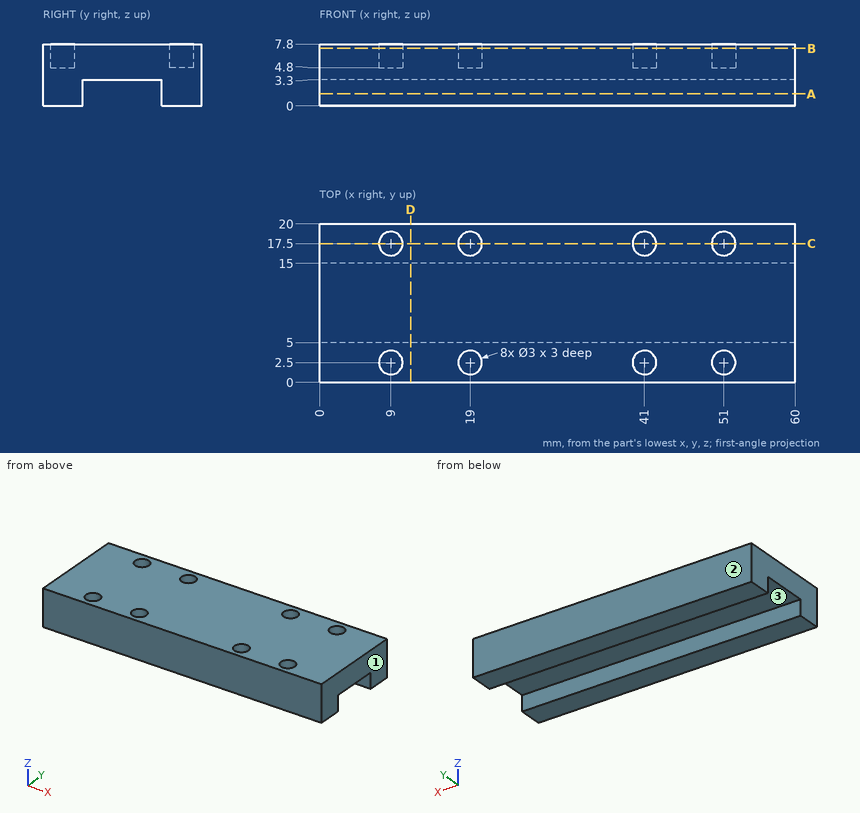
Geometry: see drawing. Coordinates: mm, zero at the bounding-box minimum. Round coordinates to 2 decimals unless told otherwise and drop trailing zeros. Write each loop counter-clockwise with the first axis right and the second up, starting at its lowest first coordinate (ties: lowest second). Pieces come first, ordered by that corner, then holes. Notation, with made-up numbers: (42, 22) -> (54, 22) arc R29 ccw to (54, 53) -> close; hole circle Ø10 at (20.25, 3). An arc over 180 degrees is marked (long way). Answer as CSV lines item,"result".
1. Mould query, pull axis Y, two halves, no side actions, for the marked faces 1, 2 and 3. Classes: +Y half, -Y half, draft (parallel to the pull), parting line (faces both ways), or undercut.
Geometry says:
face 1,"draft"
face 2,"+Y half"
face 3,"undercut"
2. Section D-D (x = 11.5). Return the cut outline in (y, z), plus the area to 3 significant figures.
Geometry says:
outline,"(0, 0) -> (5, 0) -> (5, 3.3) -> (15, 3.3) -> (15, 0) -> (20, 0) -> (20, 7.8) -> (0, 7.8) -> close"
area,"123 mm^2"
3. Section B-B (z = 7.25). Give the number of separate pieces and of enclosed holes in the cut face, plus the area to 3 significant figures.
Geometry says:
separate pieces,"1"
enclosed holes,"8"
area,"1,140 mm^2"
4. Section A-A (z = 1.5). Return the cut outline in (x, y), plus the area to 3 significant figures.
Geometry says:
outline,"(0, 0) -> (60, 0) -> (60, 5) -> (0, 5) -> close; (0, 15) -> (60, 15) -> (60, 20) -> (0, 20) -> close"
area,"600 mm^2"
5. Section C-C (y = 17.5). Return the cut outline in (x, z).
Geometry says:
outline,"(0, 0) -> (60, 0) -> (60, 7.8) -> (52.5, 7.8) -> (52.5, 4.8) -> (49.5, 4.8) -> (49.5, 7.8) -> (42.5, 7.8) -> (42.5, 4.8) -> (39.5, 4.8) -> (39.5, 7.8) -> (20.5, 7.8) -> (20.5, 4.8) -> (17.5, 4.8) -> (17.5, 7.8) -> (10.5, 7.8) -> (10.5, 4.8) -> (7.5, 4.8) -> (7.5, 7.8) -> (0, 7.8) -> close"
6. Ray query, L1, parallel to Y at x = 51, z = 5.6; L2, parallel to X at y = 2.5, z = 6.05; L3, parallel to Y at x = 22, z = 2. Return the intervals inside material, ascending. Write a range as [from, to].
Geometry says:
L1,"y = [0, 1], [4, 16], [19, 20]"
L2,"x = [0, 7.5], [10.5, 17.5], [20.5, 39.5], [42.5, 49.5], [52.5, 60]"
L3,"y = [0, 5], [15, 20]"
7. Contact query for a flat-ended pin moving along its axis: P1, Ø0.9, axis at x = 51.5, y = 2, coming from the +Z side. Output: stop coordinate, or through.
Geometry says:
P1,"stops at z = 4.8"
